```python
from build123d import *

# Parameters (mm, degrees)
F0_W     = 304.8
F0_H     = 336.55
F1_DEPTH = 12.7
F2_D     = 7.9375
F3_D     = 10.0838


with BuildPart() as f1:
    # F0 (on Top) → F1 (new body)
    with BuildSketch(Plane.XY):
        with Locations((152.4, 168.275)):
            Rectangle(F0_W, F0_H)
    extrude(amount=F1_DEPTH)

    # F2 (through all)
    with Locations(Plane(origin=(0, 0, 0), x_dir=(1, 0, 0), z_dir=(0, 0, -1))):
        with Locations((276.225, -25.4), (276.225, -311.15), (276.225, -168.275), (28.575, -168.275), (28.575, -311.15), (28.575, -25.4)):
            Hole(F2_D / 2)

    # F3 (through all)
    with Locations(Plane(origin=(0, 0, 0), x_dir=(1, 0, 0), z_dir=(0, 0, -1))):
        with Locations((231.775, -25.4), (231.775, -168.275), (231.775, -311.15), (73.025, -311.15), (73.025, -168.275), (73.025, -25.4)):
            Hole(F3_D / 2)


solid = f1.part
```
The listing builds one solid part. Answer for the finished solid, in the listing's coordinates (mm). Give positions to 0.01 mm unless a question says otherwise; leave off trailing zeros. Write each loop counter-clockwise with the first axis right and the second up, starting at its lowest first coordinate (ties: lowest second). Pieces come first, ordered by that corner, then holes. Notation, with made-up numbers: (25.25, -36) - (46.25, -36) arc R21 cw to (46.25, -4) - close; hole circle Ø11 at (45.5, 4.5). An arc over 180 degrees is marked (long way). Use one line per item in the form item = value. Start each with the question number.
1) The mould has two halves that part along Y. Classify faces 1 (the face through (150, 171, 0)), 2 (the face through (150, 0, 6)), 3 (the face through (235.491, 164.867, 6.439)): pulls with the +Y half, pulls with the -Y half, needs draft (parallel to the pull), parting line crosses it, or undercut.
2) Find section B-B on x = 28.5. Determine the outline of the cut face in (y, z), plus the area to 3 significant figures.
3) Find section A-A on y = 25.4. Determine the outline of the cut face in (x, z), plus the area to 3 significant figures.
4) Consider line 1 along X through (y, z) = (311.15, 9.25); line 2 along X through (y, z) = (30, 8.5); line 3 along Y through (x, z) = (233, 3.5). Determine where each line is inside the solid, lowest interval first. Write a range as from..to.
Geometry results:
q1.face_1 = needs draft
q1.face_2 = pulls with the -Y half
q1.face_3 = undercut
q2.outline = (0, 0) - (21.43, 0) - (21.43, 12.7) - (0, 12.7) - close; (29.37, 0) - (164.31, 0) - (164.31, 12.7) - (29.37, 12.7) - close; (172.24, 0) - (307.18, 0) - (307.18, 12.7) - (172.24, 12.7) - close; (315.12, 0) - (336.55, 0) - (336.55, 12.7) - (315.12, 12.7) - close
q2.area = 3,970 mm2
q3.outline = (0, 0) - (24.61, 0) - (24.61, 12.7) - (0, 12.7) - close; (32.54, 0) - (67.98, 0) - (67.98, 12.7) - (32.54, 12.7) - close; (78.07, 0) - (226.73, 0) - (226.73, 12.7) - (78.07, 12.7) - close; (236.82, 0) - (272.26, 0) - (272.26, 12.7) - (236.82, 12.7) - close; (280.19, 0) - (304.8, 0) - (304.8, 12.7) - (280.19, 12.7) - close
q3.area = 3,410 mm2
q4.line_1 = 0..24.61, 32.54..67.98, 78.07..226.73, 236.82..272.26, 280.19..304.8
q4.line_2 = 0..70.96, 75.09..229.71, 233.84..304.8
q4.line_3 = 0..20.51, 30.29..163.38, 173.17..306.26, 316.04..336.55
